Source: CAD feature listing. Evaluate the final solid. Frame: model axes, mm. Round coordinates to 2 decimals unless told otherwise and drop trailing zeros. Order: outer loops, then holes, each group sorted by start corner. A loop starts at its lowest first (then second) coordinate and runs counter-clockwise, first axis right, second up. Notation, with made-up numbers: M 64,68.25 L 83,68.25 A21 ccw 83,98.25 Z; hole C 84,42.25 d7. An arc over 180 degrees is marked long. Answer as CSV lines item,"result". Start each with the question number.
Item 1: Section query D-D on y = 17. Return the cut outline in (x, z) (3 decimals).
Item 2: Line query: line 1 (Y direction, x = -50.8, z = 8) (3 decimals); line 2 (X direction, y = 59.5, z = 11); line 3 (X direction, y = 49, z = 4.5). Output: solid intervals per line, ascending. Write a range as [from, to].
Item 3: First-contact query: P1, Ø4, axis at x = -63.5, y = 31.75, coming from the +Z side; P2, Ø3.5, axis at x = -0.5, y = -27, coming from the +Z side (3 decimals); P3, Ø6, axis at x = 63.5, y = -31.75, coming from the -Z side. Flat tips, straight axial feed; report the tip coordinate or a pass-through.
Item 4: Section query B-B on y = 50.8. Return the cut outline in (x, z) (3 decimals).
Item 5: Section query C-C on z = 2.25. State how many separate pieces and enclosed holes the cut face has, plus the area to 3 significant figures.
Item 6: Section query A-A on x = -50.8. Return the cut outline in (y, z) (3 decimals), plus the area to 3 significant figures.
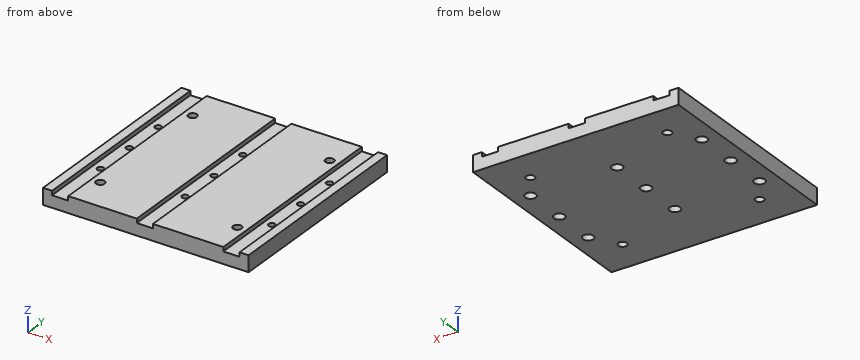
from build123d import *

# Parameters (mm, degrees)
SKETCH1_W           = 152.4
SKETCH1_H           = 152.4
SKETCH1_R           = 3.175
BOSS_EXTRUDE1_DEPTH = 12.0000014
SKETCH2_W           = 12.0000014
SKETCH2_H           = 152.4
CUT_EXTRUDE1_DEPTH  = 3.175
SKETCH3_R           = 2.38125
CUT_EXTRUDE2_DEPTH  = 109.123820917
SKETCH4_R           = 3.96875
CUT_EXTRUDE3_DEPTH  = 5.08
LPATTERN1_COUNT     = 2
LPATTERN1_PITCH     = 62.738
LPATTERN2_COUNT     = 2
LPATTERN2_PITCH     = 127


with BuildPart() as part:
    # Sketch1 → Boss-Extrude1 (new body)
    with BuildSketch(Plane.XY):
        Rectangle(SKETCH1_W, SKETCH1_H)
        with Locations((-50.8, 50.8)):
            Circle(SKETCH1_R, mode=Mode.SUBTRACT)
        with Locations((50.8, 50.8)):
            Circle(SKETCH1_R, mode=Mode.SUBTRACT)
        with Locations((50.8, -50.8)):
            Circle(SKETCH1_R, mode=Mode.SUBTRACT)
        with Locations((-50.8, -50.8)):
            Circle(SKETCH1_R, mode=Mode.SUBTRACT)
    extrude(amount=BOSS_EXTRUDE1_DEPTH)

    # Sketch2 → Cut-Extrude1 (cut)
    with BuildSketch(Plane.XY.offset(12.0000014)):
        with Locations((-63.5, 0)):
            Rectangle(SKETCH2_W, SKETCH2_H)
        with Locations((-0.6999986, 0)):
            Rectangle(SKETCH2_W, SKETCH2_H)
        with Locations((63.5, 0)):
            Rectangle(SKETCH2_W, SKETCH2_H)
    extrude(amount=-CUT_EXTRUDE1_DEPTH, mode=Mode.SUBTRACT)

    # Sketch3 → Cut-Extrude2 (cut, through all)
    with BuildSketch(Plane.XY.offset(8.8250014)):
        with Locations((-63.5, 0)):
            Circle(SKETCH3_R)
        with Locations((-63.5, 31.75)):
            Circle(SKETCH3_R)
        with Locations((-63.5, -31.75)):
            Circle(SKETCH3_R)
    cut_extrude2 = extrude(amount=-CUT_EXTRUDE2_DEPTH, mode=Mode.SUBTRACT)

    # Sketch4 → Cut-Extrude3 (cut)
    with BuildSketch(Plane(origin=(0, 0, 0), x_dir=(-1, 0, 0), z_dir=(0, 0, -1))):
        with Locations((63.5, 31.75)):
            Circle(SKETCH4_R)
        with Locations((63.5, 0)):
            Circle(SKETCH4_R)
        with Locations((63.5, -31.75)):
            Circle(SKETCH4_R)
    cut_extrude3 = extrude(amount=-CUT_EXTRUDE3_DEPTH, mode=Mode.SUBTRACT)

    # LPattern1: Cut-Extrude2, Cut-Extrude3 ×2
    with Locations(*[(i * LPATTERN1_PITCH, 0, 0) for i in range(1, LPATTERN1_COUNT)]):
        add(cut_extrude2, mode=Mode.SUBTRACT)
        add(cut_extrude3, mode=Mode.SUBTRACT)

    # LPattern2: Cut-Extrude2, Cut-Extrude3 ×2
    with Locations(*[(i * LPATTERN2_PITCH, 0, 0) for i in range(1, LPATTERN2_COUNT)]):
        add(cut_extrude2, mode=Mode.SUBTRACT)
        add(cut_extrude3, mode=Mode.SUBTRACT)


solid = part.part
Results:
1,outline,"M -76.2,0 L 76.2,0 L 76.2,12 L 69.5,12 L 69.5,8.825 L 57.5,8.825 L 57.5,12 L 5.3,12 L 5.3,8.825 L -6.7,8.825 L -6.7,12 L -57.5,12 L -57.5,8.825 L -69.5,8.825 L -69.5,12 L -76.2,12 Z"
2,line 1,"[-76.2, -53.975], [-47.625, 47.625], [53.975, 76.2]"
2,line 2,"[-76.2, -69.5], [-57.5, -6.7], [5.3, 57.5], [69.5, 76.2]"
2,line 3,"[-76.2, -53.42], [-48.18, 48.18], [53.42, 76.2]"
3,P1,"through"
3,P2,"z = 8.825"
3,P3,"z = 5.08"
4,outline,"M -76.2,0 L -53.975,0 L -53.975,12 L -57.5,12 L -57.5,8.825 L -69.5,8.825 L -69.5,12 L -76.2,12 Z; M -47.625,0 L 47.625,0 L 47.625,12 L 5.3,12 L 5.3,8.825 L -6.7,8.825 L -6.7,12 L -47.625,12 Z; M 53.975,0 L 76.2,0 L 76.2,12 L 69.5,12 L 69.5,8.825 L 57.5,8.825 L 57.5,12 L 53.975,12 Z"
5,separate pieces,"1"
5,enclosed holes,"13"
5,area,"22,700 mm^2"
6,outline,"M -76.2,0 L -53.975,0 L -53.975,12 L -76.2,12 Z; M -47.625,0 L 47.625,0 L 47.625,12 L -47.625,12 Z; M 53.975,0 L 76.2,0 L 76.2,12 L 53.975,12 Z"
6,area,"1,680 mm^2"
